from build123d import *

# Parameters (mm, degrees)
SKETCH1_R           = 10.16
BOSS_EXTRUDE1_DEPTH = 5.588
SKETCH3_R           = 8.128
CUT_EXTRUDE1_DEPTH  = 10.16
SKETCH4_R           = 8.763
CUT_EXTRUDE2_DEPTH  = 1.016


with BuildPart() as part:
    # Sketch1 → Boss-Extrude1 (new body)
    with BuildSketch(Plane(origin=(0, 0, 0), x_dir=(1, 0, 0), z_dir=(0, 1, 0))):
        Circle(SKETCH1_R)
    extrude(amount=BOSS_EXTRUDE1_DEPTH)

    # Sketch2 → Cut-Revolve1 (revolve, cut)
    with BuildSketch(Plane.XY):
        with BuildLine():
            Line((-10.16, 4.191), (-10.16, 1.397))
            ThreePointArc((-10.16, 1.397), (-8.763, 2.794), (-10.16, 4.191))
        make_face()
    revolve(axis=Axis((0, 5.588, 0), (0, -1, 0)), mode=Mode.SUBTRACT)

    # Sketch3 → Cut-Extrude1 (cut)
    with BuildSketch(Plane(origin=(0, 5.588, 0), x_dir=(1, 0, 0), z_dir=(0, 1, 0))):
        Circle(SKETCH3_R)
    extrude(amount=-CUT_EXTRUDE1_DEPTH, mode=Mode.SUBTRACT)

    # Sketch4 → Cut-Extrude2 (cut)
    with BuildSketch(Plane(origin=(0, 5.588, 0), x_dir=(1, 0, 0), z_dir=(0, 1, 0))):
        Circle(SKETCH4_R)
    extrude(amount=-CUT_EXTRUDE2_DEPTH, mode=Mode.SUBTRACT)


solid = part.part
The model under review builds one solid part; all positions refer to its coordinate system, in mm. A direction names the side the tool comes from. Round coordinates to 2 decimals unless told otherwise and drop trailing zeros. Write each loop counter-clockwise with the first axis right and the second up, starting at its lowest first coordinate (ties: lowest second). Pieces come first, ordered by that corner, then holes. Notation, with made-up numbers: M 89,89.5 L 101,89.5 A19 cw 101,119.5 Z; hole C 88.25,2.5 d3. An arc over 180 degrees is marked long. Answer as CSV lines item,"result". Start each with the question number.
Q1. Wall thickness on line 1 along X through (y, z) = (5.35, 0); line 2 along X through (y, z) = (2.7, 0); line 3 along Y through (x, z) = (2, -8.5): over which ranges is each line inside the solid? List them lowest first.
Q2. Tool access review of faces 1 (the face through (-5, 0, -7)), 2 (the face through (8, 4.572, 3)): name each direction out of +Z, -Z, +X, -X, +Y, -Y from which nothing blocks a thin tool from reaching the whole face with its end or side.
Q3. Clearance check with flat-ended pins moving along their axes: P1, Ø3, axis at x = 5.5, y = 0.5, coming from the -Z side; P2, Ø3, axis at x = -2, y = 3, coming from the -Z side; P3, Ø2, axis at x = 4.5, z = -2.5, coming from the -Y side. State where each tip first meets the part, or that it passes through.
Q4. The part is to be moulded in two halves that separate along Z. For faces 3 (the face through (-8, 5.588, 4)), 4 (the face through (-1.323, 0.689, -10.074)), 5 (the face through (8.36, 5.09, -2.63)), say which applies: +Z half, -Z half, draft (parallel to the pull), parting line (faces both ways), or undercut.
Q5. Consider section C-C, the plane y = 3.1. Give the boundary of the cut face in (x, z), then the cut area to 3 significant figures.
Result set:
1,line 1,"x = -10.16 to -8.76, 8.76 to 10.16"
1,line 2,"x = -8.77 to -8.13, 8.13 to 8.77"
1,line 3,"y = 0 to 4.57"
2,face 1,"+Z, -Z, +X, -X, -Y"
2,face 2,"+Y"
3,P1,"stops at z = -9.34"
3,P2,"stops at z = -10.1"
3,P3,"passes through"
4,face 3,"draft"
4,face 4,"parting line"
4,face 5,"undercut"
5,outline,"C 0,0 d17.59; hole C 0,0 d16.26"
5,area,"35.6 mm²"
